```python
from build123d import *

# Parameters (mm, degrees)
BOSS_EXTRUDE1_DEPTH   = 8
BOSS_EXTRUDE1_2_DEPTH = 8
BOSS_EXTRUDE2_DEPTH   = 8


with BuildPart() as part:
    # Sketch1 → Boss-Extrude1 (new body)
    with BuildSketch(Plane.XY):
        with BuildLine():
            Line((-2.974906864, -18.61376988), (-2.974906864, -12.809076046))
            ThreePointArc((-2.974906864, -12.809076046), (-5.875216569, -11.764536976), (-8.452657067, -10.073484427))
            ThreePointArc((-8.452657067, -10.073484427), (-12.467828418, -10.424766402), (-12.116546443, -14.439937753))
            ThreePointArc((-12.116546443, -14.439937753), (-7.828997981, -17.14728231), (-2.974906864, -18.61376988))
        make_face()
    extrude(amount=BOSS_EXTRUDE1_DEPTH)



with BuildPart() as body_2:
    # Sketch1 → Boss-Extrude1 2 (new body)
    with BuildSketch(Plane.XY):
        with BuildLine():
            ThreePointArc((8.452657067, -10.073484427), (5.898262695, -11.752999497), (3.025093136, -12.797316575))
            Line((3.025093136, -12.797316575), (3.025093136, -18.60567955))
            ThreePointArc((3.025093136, -18.60567955), (7.852112038, -17.136710202), (12.116546443, -14.439937753))
            ThreePointArc((12.116546443, -14.439937753), (12.467828418, -10.424766402), (8.452657067, -10.073484427))
        make_face()
    extrude(amount=BOSS_EXTRUDE1_2_DEPTH)


with BuildPart() as part_1:
    add(part.part)

    add(body_2.part)  # Boss-Extrude2 merges body 2
    # Sketch2 → Boss-Extrude2 (add)
    with BuildSketch(Plane(origin=(0, 0, 0), x_dir=(-1, 0, 0), z_dir=(0, 0, -1))):
        with BuildLine():
            Line((-3.025093136, -15.711422963), (-3.025093136, -12.797316575))
            Line((-3.025093136, -12.797316575), (-3.025093136, -9.53146429))
            ThreePointArc((-3.025093136, -9.53146429), (-4.818177628, -8.762714439), (-6.427876097, -7.660444431))
            ThreePointArc((-6.427876097, -7.660444431), (-14.880868414, -8.399985432), (-14.141327413, -16.852977749))
            ThreePointArc((-14.141327413, -16.852977749), (0, -22), (14.141327413, -16.852977749))
            ThreePointArc((14.141327413, -16.852977749), (14.880868414, -8.399985432), (6.427876097, -7.660444431))
            ThreePointArc((6.427876097, -7.660444431), (4.795110846, -8.775358225), (2.974906864, -9.547247203))
            Line((2.974906864, -9.547247203), (2.974906864, -12.809076046))
            ThreePointArc((2.974906864, -12.809076046), (5.875216569, -11.764536976), (8.452657067, -10.073484427))
            ThreePointArc((8.452657067, -10.073484427), (12.467828418, -10.424766402), (12.116546443, -14.439937753))
            ThreePointArc((12.116546443, -14.439937753), (7.828997981, -17.14728231), (2.974906864, -18.61376988))
            Line((2.974906864, -18.61376988), (2.974906864, -15.711422963))
            ThreePointArc((2.974906864, -15.711422963), (-0.025093136, -18.711422963), (-3.025093136, -15.711422963))
        make_face()
        with BuildLine():
            ThreePointArc((12.116546443, -14.439937753), (12.467828418, -10.424766402), (8.452657067, -10.073484427))
            ThreePointArc((8.452657067, -10.073484427), (5.875216569, -11.764536976), (2.974906864, -12.809076046))
            Line((2.974906864, -12.809076046), (2.974906864, -18.61376988))
            ThreePointArc((2.974906864, -18.61376988), (7.828997981, -17.14728231), (12.116546443, -14.439937753))
        make_face()
    extrude(amount=BOSS_EXTRUDE2_DEPTH)


solid = part_1.part
```
Model file for the job. Use its own axes, mm. A direction names the side the tool comes from. Coordinates: 2 decimals unless noted, no trailing zeros. Write each loop counter-clockwise with the first axis right and the second up, starting at its lowest first coordinate (ties: lowest second). Pieces come first, ordered by that corner, then holes. Notation, with made-up numbers: (81, 54.5) - (102, 54.5) arc R20 ccw to (102, 84.5) - close; hole circle Ø9 at (-10, -15.5). An arc over 180 degrees is marked (long way). Use a Markdown table: item, result. Add a question column.
Item 1: 3-axis set-ups, long thin cutter, end or side, ignore diameter. For faces 4 (the face through (3.025, -14, 0)), 5 (the face through (-4.82, -8.76, -3.94)), 6 (the face through (12.508, -10.473, 3.944)), 7 (the face through (-7.89, -17.12, 3.94)): which of +Z, -Z, +X, -X, +Y, -Y reach the whole face in a straight line?
Item 2: Drill centre lines: line 1 along Z through (x, y) = (-14, -15); line 2 along X through (y, z) = (-16.5, 6.5); line 3 along X through (y, z) = (-15.5, -5). Where is each one in solid material? Low to high.
Item 3: Band-saw the part on A-A, the plane z = 5. Write the cut outline in (x, y).
Item 4: Two-plate mould, pull along X, no slides. Class faces 1 (the face through (7.788, -17.166, 3.944)), 2 (the face through (8, -14, 8)), 3 (the face through (-0.04, -18.71, -3.94)): pulls with the +X half, pulls with the -X half, needs draft (parallel to the pull), parting line crosses it, or undercut.
Item 5: Drop flat-ended pins along their axis: pin 1 (1 mm diameter, centred on x = 6, z = -0.5, fed in from -Y); pin 2 (4.5 mm diameter, centred on y = -14.5, z = 3.5, fed in from -X); pin 3 (2 mm diameter, centred on x = -4, z = 4, fed in from +Y); pin 4 (4.5 mm diameter, centred on x = -7.5, y = -17.5, fed in from +Z). Give the stop position or say it passes through.
Item 6: Band-saw the part on D-D, the plane x = -4. Write the cut outline in (y, z), and give its area (3 significant figures).
Item 7: Band-saw the part on B-B, the plane y = -8.25. Write the cut outline in (x, z), and give its area (3 significant figures).
A:
| question | item | result |
|---|---|---|
| 1 | face 4 | +Z, +Y |
| 1 | face 5 | +Z, -Z, +Y |
| 1 | face 6 | +Z |
| 1 | face 7 | +Z, -X, -Y |
| 2 | line 1 | z = -8 to 0 |
| 2 | line 2 | x = -9.11 to -2.97, 3.03 to 9.11 |
| 2 | line 3 | x = -15.33 to -2.97, 3.03 to 15.33 |
| 3 | outline | (-12.12, -14.44) arc R18.85 ccw to (-2.97, -18.61) - (-2.97, -12.81) arc R13.15 cw to (-8.45, -10.07) arc R2.85 ccw to start; (3.03, -18.61) arc R18.85 ccw to (12.12, -14.44) arc R2.85 ccw to (8.45, -10.07) arc R13.15 cw to (3.03, -12.8) - close |
| 4 | face 1 | pulls with the +X half |
| 4 | face 2 | needs draft |
| 4 | face 3 | undercut |
| 5 | pin 1 | stops at y = -21.3 |
| 5 | pin 2 | stops at x = -13.13 |
| 5 | pin 3 | stops at y = -12.16 |
| 5 | pin 4 | stops at z = 8 |
| 6 | outline | (-21.63, -8) - (-9.17, -8) - (-9.17, 0) - (-12.53, 0) - (-12.53, 8) - (-18.42, 8) - (-18.42, 0) - (-21.63, 0) - close |
| 6 | area | 147 mm² |
| 7 | outline | (-14.75, -8) - (-5.65, -8) - (-5.65, 0) - (-14.75, 0) - close; (5.65, -8) - (14.75, -8) - (14.75, 0) - (5.65, 0) - close |
| 7 | area | 146 mm² |
